Study the drawing (mm; zero at the part's minimum x, y, z) and answer. Round coordinates to 2 decimals unless told otherwise and drop trailing zeros. Loops run counter-clockwise (first coordinate to the right, second up) from the corner with the lowest first, then second, coordinate; pieces in that order, holes last. Notation, with made-up numbers: M -37.75,41.25 L 12.25,41.25 A14 cw 12.25,47.25 Z; hole C -9.75,21 d2. An arc over 180 degrees is marked long. Put each result on its own line as item: value. Start each with the question number.
(1) Flat-ended cylindrical pins translate along their axes: P1, Ø1.5, axis at y = 0.5, z = 1.5, coming from the -X side; P2, Ø7.5, axis at x = 8.15, z = 6.11, coming from the -Y side. Find the tip coordinate at first contact, or state that the pin passes through.
(2) Section D-D, the plane z = 12.25 is taken. Determine the outline of the cut face in (x, y), then the cut area to 3 significant figures.
(3) Determine the mould class of the marked faces 1, 2 and 3 for opening direction X: released by +X, released by -X, zero draft, split by the parting line, or undercut.
(4) Straight lines are drawn through the part: line 1 (X direction, y = 1.2, z = 6); line 2 (Z direction, x = 8.15, y = 1.85); line 3 (X direction, y = 1.7, z = 7.75). For each, find the intervals that lie inside material, in ascending order.
(5) Section C-C, the plane x = 8.15 is taken. Determine the outline of the cut face in (y, z).
(6) Section B-B, the plane y = 2.4 is taken. Determine the outline of the cut face in (x, z).
(7) Section A-A, the plane z = 6.75 is taken. Determine the outline of the cut face in (x, y), then the cut area to 3 significant figures.
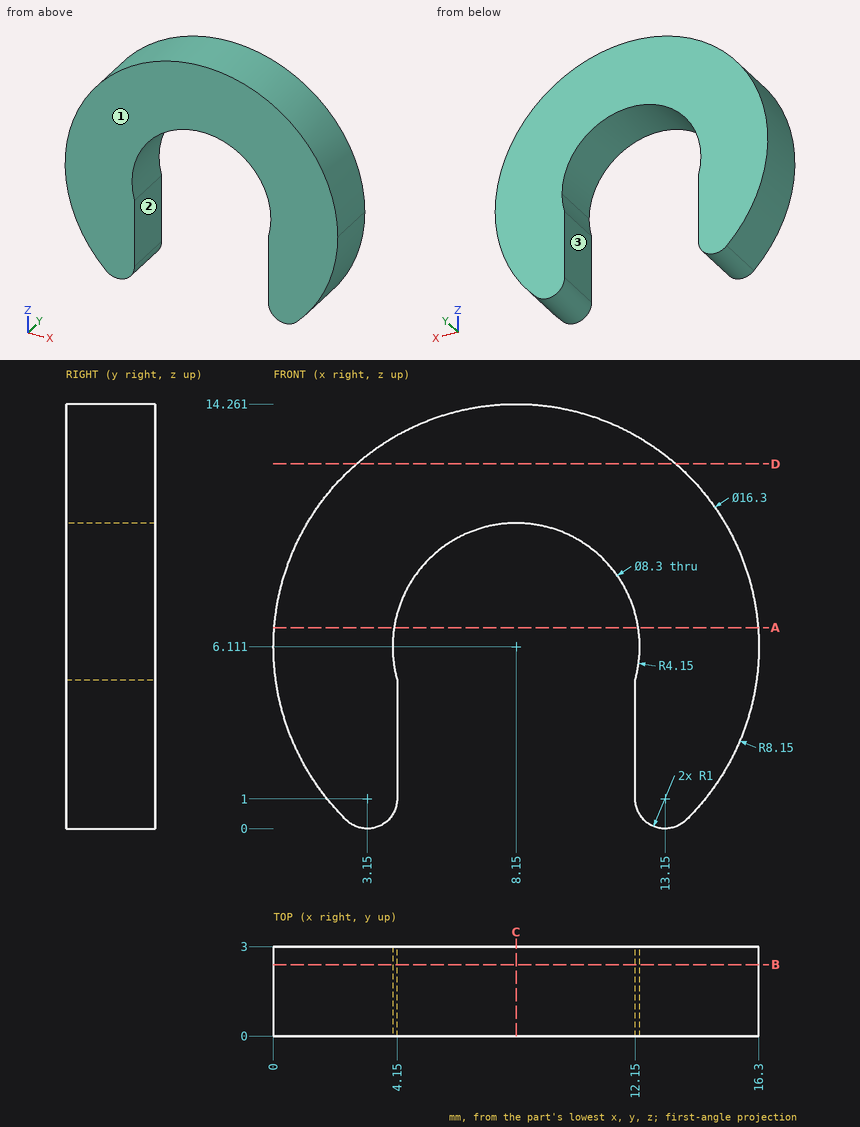
Recorded:
1. P1: stops at x = 0.97
1. P2: passes through
2. outline: M 2.79,0 L 13.51,0 L 13.51,3 L 2.79,3 Z
2. area: 32.2 mm²
3. face 1: zero draft
3. face 2: undercut
3. face 3: undercut
4. line 1: x = 0 to 4, 12.3 to 16.3
4. line 2: z = 10.26 to 14.26
4. line 3: x = 0.17 to 4.34, 11.96 to 16.13
5. outline: M 0,10.26 L 3,10.26 L 3,14.26 L 0,14.26 Z
6. outline: M 2.45,0.29 A1 ccw 4.15,1 L 4.15,5.01 A4.15 cw long 12.15,5.01 L 12.15,1 A1 ccw 13.85,0.29 A8.15 ccw long Z
7. outline: M 0.03,0 L 4.05,0 L 4.05,3 L 0.03,3 Z; M 12.25,0 L 16.27,0 L 16.27,3 L 12.25,3 Z
7. area: 24.1 mm²
